from build123d import *

# Parameters (mm, degrees)
MEASURED_PCB_37X37_W                                = 37
MEASURED_PCB_37X37_H                                = 37
PCB_VISUAL_THICKNESS_1MM_UNMEASURED_DEPTH           = 1
LENS_HEIGHT25_FROM_PCB_FRONT_START                  = 1
LENS_OD13_CENTER_PROVISIONAL_R                      = 6.5
LENS_HEIGHT25_FROM_PCB_FRONT_DEPTH                  = 25
FOUR_MEASURED_D2_HOLES_PROVISIONAL_LOCAT_DEPTH      = 37.884956283
FOUR_MEASURED_D2_HOLES_PROVISIONAL_LOCAT_DEPTH_BACK = 37.884956283
HOLE_CENTERS33_PROVISIONAL_R                        = 1


with BuildPart() as part:
    # Measured_PCB_37x37 → PCB_visual_thickness_1mm_UNMEASURED (new body)
    with BuildSketch(Plane.XY):
        Rectangle(MEASURED_PCB_37X37_W, MEASURED_PCB_37X37_H)
    extrude(amount=PCB_VISUAL_THICKNESS_1MM_UNMEASURED_DEPTH)

    # Lens_OD13_center_PROVISIONAL → Lens_height25_from_PCB_front (add)
    with BuildSketch(Plane.XY.offset(LENS_HEIGHT25_FROM_PCB_FRONT_START)):
        Circle(LENS_OD13_CENTER_PROVISIONAL_R)
    extrude(amount=LENS_HEIGHT25_FROM_PCB_FRONT_DEPTH)

    # Hole_centers33_PROVISIONAL → Four_measured_D2_holes_PROVISIONAL_locations (cut, two sides: drawn at the far end of the back side and taken through both)
    with BuildSketch(Plane.XY.offset(-FOUR_MEASURED_D2_HOLES_PROVISIONAL_LOCAT_DEPTH_BACK)):
        with Locations((-16.5, -16.5)):
            Circle(HOLE_CENTERS33_PROVISIONAL_R)
        with Locations((-16.5, 16.5)):
            Circle(HOLE_CENTERS33_PROVISIONAL_R)
        with Locations((16.5, -16.5)):
            Circle(HOLE_CENTERS33_PROVISIONAL_R)
        with Locations((16.5, 16.5)):
            Circle(HOLE_CENTERS33_PROVISIONAL_R)
    extrude(amount=FOUR_MEASURED_D2_HOLES_PROVISIONAL_LOCAT_DEPTH + FOUR_MEASURED_D2_HOLES_PROVISIONAL_LOCAT_DEPTH_BACK, mode=Mode.SUBTRACT)


solid = part.part
Model file for the job. Use its own axes, mm. A direction names the side the tool comes from. Round coordinates to 2 decimals unless told otherwise and drop trailing zeros. Order: outer loops, then holes, each group sorted by start corner. A loop starts at its lowest first (then second) coordinate and runs counter-clockwise, first axis right, second up. Notation, with made-up numbers: M 0.25,15.25 L 48.25,15.25 A21 ccw 48.25,26.25 Z; hole C -19.75,16 d3. An arc over 180 degrees is marked long. Write each question's results on one line, items separated by ' | '. Start each with the question number.
(1) Saw through at A-A, the plane y = -16.5. Give the cut face in (x, z), then the cut area to 3 significant figures.
(2) Two-plate mould, pull along Y, no slides. Class faces 3 (the face through (-0.3, -18.5, 0.5)), 4 (the face through (-8, 0, 1)), 5 (the face through (-16.04, 15.61, 0.49)), 6 (the face through (16.96, -17.39, 0.49)): pulls with the +Y half, pulls with the -Y half, needs draft (parallel to the pull), parting line crosses it, or undercut.
(3) Which spindle directions (+Z, -Z, +X, -X, +Y, -Y) get a long thin tool onto all of the face, cutting with end or side? Do faces 1 (the face through (-5.158, -3.955, 13.325)), 2 (the face through (-0.3, 18.5, 0.5)). Say none if no direction does.
(4) Drop flat-ended pins along their axis: pin 1 (6 mm diameter, centred on x = 1.5, z = 13.5, fed in from +Y); pin 2 (6 mm diameter, centred on x = -7, y = 10.5, fed in from +Z); pin 3 (10 mm diameter, centred on x = -9.5, z = 17.5, fed in from +Y); pin 4 (1.8 mm diameter, centred on x = -16.5, y = 16.5, fed in from +Z). Give the stop position or say it passes through.
(5) Probe probe 1 along Y at (x, z) = (16.5, 0.2); probe 2 along Z at (x, y) = (-16, -15); probe 3 along Y at (x, z) = (3, 19.25). List the from-to ranges inside material, lowest first. Write a range as from..to.
(6) Saw through at C-C, the plane x = 0. Give the cut face in (y, z).
Established:
1) outline: M -18.5,0 L -17.5,0 L -17.5,1 L -18.5,1 Z; M -15.5,0 L 15.5,0 L 15.5,1 L -15.5,1 Z; M 17.5,0 L 18.5,0 L 18.5,1 L 17.5,1 Z | area: 33.0 mm^2
2) face 3: pulls with the -Y half | face 4: needs draft | face 5: undercut | face 6: undercut
3) face 1: +Z | face 2: +Z, -Z, +X, -X, +Y
4) pin 1: stops at y = 6.5 | pin 2: stops at z = 1 | pin 3: stops at y = 4.69 | pin 4: passes through
5) probe 1: y = -18.5..-17.5, -15.5..15.5, 17.5..18.5 | probe 2: z = 0..1 | probe 3: y = -5.77..5.77
6) outline: M -18.5,0 L 18.5,0 L 18.5,1 L 6.5,1 L 6.5,26 L -6.5,26 L -6.5,1 L -18.5,1 Z
